from build123d import *

# Parameters (mm, degrees)
SKETCH2_R           = 4.7625
SKETCH2_R_2         = 12.8
BOSS_EXTRUDE2_DEPTH = 5.334
SKETCH3_R           = 6.35
SKETCH3_R_2         = 4.7625
CUT_EXTRUDE3_DEPTH  = 2.667
SKETCH3_2_R         = 4.7625
CUT_EXTRUDE4_DEPTH  = 6.334


with BuildPart() as part:
    # Sketch2 → Boss-Extrude2 (new body)
    with BuildSketch(Plane.XY):
        Polygon((-55.022779977, 2.330692017), (-24, -20.208676973), (24, -20.208676973), (55.022779977, 2.330692017), (34.005948181, 67.013849238), (-34.005948181, 67.013849238), align=None)
        Circle(SKETCH2_R, mode=Mode.SUBTRACT)
        with Locations((-24, 20.208676973)):
            Circle(SKETCH2_R_2, mode=Mode.SUBTRACT)
        with Locations((24, 20.208676973)):
            Circle(SKETCH2_R_2, mode=Mode.SUBTRACT)
        with Locations((24, 51.583676973)):
            Circle(SKETCH2_R_2, mode=Mode.SUBTRACT)
    extrude(amount=BOSS_EXTRUDE2_DEPTH)

    # Sketch3 → Cut-Extrude3 (cut)
    with BuildSketch(Plane.XY.offset(5.334)):
        Circle(SKETCH3_R)
        Circle(SKETCH3_R_2, mode=Mode.SUBTRACT)
        with Locations((45.751679669, 9.848845061)):
            Circle(SKETCH3_R)
        with Locations((45.751679669, 9.848845061)):
            Circle(SKETCH3_R_2, mode=Mode.SUBTRACT)
        with Locations((0, 33.008676973)):
            Circle(SKETCH3_R)
        with Locations((0, 33.008676973)):
            Circle(SKETCH3_R_2, mode=Mode.SUBTRACT)
        with Locations((-45.751679669, 9.848845061)):
            Circle(SKETCH3_R)
        with Locations((-45.751679669, 9.848845061)):
            Circle(SKETCH3_R_2, mode=Mode.SUBTRACT)
    extrude(amount=-CUT_EXTRUDE3_DEPTH, mode=Mode.SUBTRACT)

    # Sketch3_2 → Cut-Extrude4 (cut, through all)
    with BuildSketch(Plane.XY.offset(5.334)):
        with Locations((-45.751679669, 9.848845061)):
            Circle(SKETCH3_2_R)
        with Locations((0, 33.008676973)):
            Circle(SKETCH3_2_R)
        with Locations((45.751679669, 9.848845061)):
            Circle(SKETCH3_2_R)
    extrude(amount=-CUT_EXTRUDE4_DEPTH, mode=Mode.SUBTRACT)


solid = part.part
Here's how the part is built. I have some questions about the finished solid (model axes, mm). A direction names the side the tool comes from. Coordinates: 2 decimals unless noted, no trailing zeros. Write each loop counter-clockwise with the first axis right and the second up, starting at its lowest first coordinate (ties: lowest second). Pieces come first, ordered by that corner, then holes.
Item 1: Will these pins go through, and if not, where does the flat tip stop? pin 1 (6.5 mm diameter, centred on x = -46, y = 10, fed in from +Z); pin 2 (10 mm diameter, centred on x = -45.75, y = 9.85, fed in from +Z); pin 3 (3 mm diameter, centred on y = 4.5, z = 1.5, fed in from +X).
Item 2: I want a section at A-A on x = 0. Write out the boundary of the cut face in (y, z), and give its area (3 significant figures).
Item 3: On a 3-axis mill with a long thin cutter (end or side, diameter ignored), from which of +Z, -Z, +X, -X, +Y, -Y can I reach the whole of each face in a straight line? I mean faces 1 (the cylindrical face through (-34.16, 12.42, 2.63)), 2 (the cylindrical face through (-1.38, -6.2, 4.02)). Say none if no direction works.
Item 4: I want a section at D-D on y = 23. Write out the boundary of the cut face in (x, z), and give its area (3 significant figures).
Item 5: I want a section at B-B on y = 40.5. Write out the boundary of the cut face in (x, z).
Item 6: If I drill on line 1 (Y direction, x = 24, z = 3.1); line 2 (X direction, y = 21, z = 4.15); line 3 (Y direction, x = 14, z = 2.95), over which ranges is the centre line in solid material (lowest first)?
Item 7: I want a section at C-C on x = -45. Write out the boundary of the cut face in (y, z), and give its area (3 significant figures).
Item 8: If we mould it in two halves opening along Y, with no side actions, what happens to faces 3 (the flat face through (0, -20.209, 3)), 4 (the cylindrical face through (-1.03, 28.36, 1.35)), 5 (the flat face through (0, 67.014, 3))? For each: +Y half, -Y half, draft (parallel to the pull), parting line (faces both ways), or undercut.
Findings below:
1. pin 1: passes through
1. pin 2: stops at z = 2.67
1. pin 3: stops at x = 54.81
2. outline: (-20.21, 0) - (-4.76, 0) - (-4.76, 2.67) - (-6.35, 2.67) - (-6.35, 5.33) - (-20.21, 5.33) - close; (4.76, 0) - (28.25, 0) - (28.25, 2.67) - (26.66, 2.67) - (26.66, 5.33) - (6.35, 5.33) - (6.35, 2.67) - (4.76, 2.67) - close; (37.77, 0) - (67.01, 0) - (67.01, 5.33) - (39.36, 5.33) - (39.36, 2.67) - (37.77, 2.67) - close
2. area: 347 mm2
3. face 1: +Z, -Z
3. face 2: +Z
4. outline: (-48.31, 0) - (-36.49, 0) - (-36.49, 5.33) - (-48.31, 5.33) - close; (-11.51, 0) - (11.51, 0) - (11.51, 5.33) - (-11.51, 5.33) - close; (36.49, 0) - (48.31, 0) - (48.31, 5.33) - (36.49, 5.33) - close
4. area: 249 mm2
5. outline: (-42.62, 0) - (17.6, 0) - (17.6, 5.33) - (-42.62, 5.33) - close; (30.4, 0) - (42.62, 0) - (42.62, 5.33) - (30.4, 5.33) - close
6. line 1: y = -20.21 to 7.41, 33.01 to 38.78, 64.38 to 67.01
6. line 2: x = -48.96 to -36.78, -11.22 to 11.22, 36.78 to 48.96
6. line 3: y = -20.21 to 12.22, 28.2 to 43.59, 59.57 to 67.01
7. outline: (-4.95, 0) - (5.15, 0) - (5.15, 2.67) - (3.54, 2.67) - (3.54, 5.33) - (-4.95, 5.33) - close; (14.55, 0) - (33.18, 0) - (33.18, 5.33) - (16.15, 5.33) - (16.15, 2.67) - (14.55, 2.67) - close
7. area: 145 mm2
8. face 3: -Y half
8. face 4: undercut
8. face 5: +Y half
